Geometry check sheet. Reference: the model listing, model coordinates, mm. A direction names the side the tool comes from. Round coordinates to 2 decimals unless told otherwise and drop trailing zeros. Loops run counter-clockwise (first coordinate to the right, second up) from the corner with the lowest first, then second, coordinate; pieces in that order, holes last. Notation, with made-up numbers: M 21.5,-21.5 L 37.5,-21.5 A16 cw 37.5,8.5 Z; hole C 22.25,55.5 d1. An arc over 180 degrees is marked long. Write item = value, one per line.
from build123d import *

# Parameters (mm, degrees)
SKETCH_1_W      = 120
SKETCH_1_H      = 90
SKETCH_1_R      = 1.65
SKETCH_1_R_2    = 2
SKETCH_1_W_2    = 50
SKETCH_1_H_2    = 35
EXTRUDE_1_DEPTH = 5
FILLET_1_R      = 5
FILLET_2_R      = 5


with BuildPart() as part:
    # 草图1 → 凸台-拉伸1 (new body)
    with BuildSketch(Plane.XY):
        with Locations((-60, -45)):
            Rectangle(SKETCH_1_W, SKETCH_1_H)
        with Locations((-115, -85)):
            Circle(SKETCH_1_R, mode=Mode.SUBTRACT)
        with Locations((-5, -85)):
            Circle(SKETCH_1_R, mode=Mode.SUBTRACT)
        with Locations((-5, -5)):
            Circle(SKETCH_1_R, mode=Mode.SUBTRACT)
        with Locations((-115, -5)):
            Circle(SKETCH_1_R, mode=Mode.SUBTRACT)
        with Locations((-24.95, -45)):
            Circle(SKETCH_1_R_2, mode=Mode.SUBTRACT)
        with Locations((-35.215907319, -69.784092681)):
            Circle(SKETCH_1_R_2, mode=Mode.SUBTRACT)
        with Locations((-60, -80.05)):
            Circle(SKETCH_1_R_2, mode=Mode.SUBTRACT)
        with Locations((-84.784092681, -69.784092681)):
            Circle(SKETCH_1_R_2, mode=Mode.SUBTRACT)
        with Locations((-84.784092681, -20.215907319)):
            Circle(SKETCH_1_R_2, mode=Mode.SUBTRACT)
        with Locations((-60, -9.95)):
            Circle(SKETCH_1_R_2, mode=Mode.SUBTRACT)
        with Locations((-35.215907319, -20.215907319)):
            Circle(SKETCH_1_R_2, mode=Mode.SUBTRACT)
        with Locations((-75, -45)):
            Rectangle(SKETCH_1_W_2, SKETCH_1_H_2, mode=Mode.SUBTRACT)
    extrude(amount=EXTRUDE_1_DEPTH)

    # 圆角1
    fillet_1_edges = [part.edges().sort_by_distance(p)[0] for p in [
        (0, -90, 2.5),
        (-120, -90, 2.5),
        (-120, 0, 2.5),
        (0, 0, 2.5),
    ]]
    fillet(fillet_1_edges, radius=FILLET_1_R)

    # 圆角2
    fillet_2_edges = [part.edges().sort_by_distance(p)[0] for p in [
        (-100, -27.5, 2.5),
        (-100, -62.5, 2.5),
        (-50, -62.5, 2.5),
        (-50, -27.5, 2.5),
    ]]
    fillet(fillet_2_edges, radius=FILLET_2_R)


solid = part.part
(1) Sectioned sample at C-C on x = -93. Record the cut outline in (y, z).
Result set:
outline = M -90,0 L -62.5,0 L -62.5,5 L -90,5 Z; M -27.5,0 L 0,0 L 0,5 L -27.5,5 Z
(2) Sectioned sample at D-D on z = 3. State how many separate pieces and enclosed holes the cut face has, then the cut area to 3 significant figures.
Result set:
separate_pieces = 1
enclosed_holes = 12
area = 8,930 mm2
(3) Depth check by flat-ended pin: pin 1 Ø4.5 at (x, y) = (-60, -80.05) entering from -Z; pin 2 Ø2.5 at (x, y) = (-5, -5) entering from +Z. Enter the tip coordinate at first touch or a pass-through.
Result set:
pin_1 = 0
pin_2 = through
(4) Tool access check on faces 1 (the flat face through (-50, -45, 2)), 2 (the flat face through (-48, -44, 0)). Record the directions out of +Z, -Z, +X, -X, +Y, -Y that give a thin tool (end or side, any length) a straight path to the whole face; none if there is none.
Result set:
face_1 = +Z, -Z
face_2 = -Z, +X, -X, +Y, -Y
(5) Release check for a two-part mould opening along X. For faces 3 (the cylindrical face through (-60.26, -78.067, 2.465)), 4 (the cylindrical face through (-2, -1, 3)), 5 (the flat face through (-61, -90, 2)) record: released by +X, released by -X, zero draft, split by the parting line, or undercut.
Result set:
face_3 = undercut
face_4 = released by +X
face_5 = zero draft
(6) Sectioned sample at B-B on x = -60. Record the cut outline in (y, z), then the cut area to 3 significant figures.
Result set:
outline = M -90,0 L -82.05,0 L -82.05,5 L -90,5 Z; M -78.05,0 L -62.5,0 L -62.5,5 L -78.05,5 Z; M -27.5,0 L -11.95,0 L -11.95,5 L -27.5,5 Z; M -7.95,0 L 0,0 L 0,5 L -7.95,5 Z
area = 235 mm2
(7) Sectioned sample at A-A on y = -80.05. Record the cut outline in (x, z), then the cut area to 3 significant figures.
Result set:
outline = M -120,0 L -62,0 L -62,5 L -120,5 Z; M -58,0 L 0,0 L 0,5 L -58,5 Z
area = 580 mm2
(8) Material ranges on line 1 along Y through (x, z) = (-115, 2.2); line 2 along Y through (x, z) = (-95.5, 3.3); line 3 along X through (y, z) = (-68, 1.05), recorded low to high. Write a range as from..to.
Result set:
line_1 = -90..-86.65, -83.35..-6.65, -3.35..0
line_2 = -90..-62.47, -27.53..0
line_3 = -120..-85.69, -83.88..-36.12, -34.31..0
